from build123d import *

# Parameters (mm, degrees)
SKETCH1_W           = 8
SKETCH1_H           = 23
BOSS_EXTRUDE1_DEPTH = 3
SKETCH2_W           = 8
SKETCH2_H           = 3
BOSS_EXTRUDE2_DEPTH = 18
SKETCH3_R           = 1.75
CUT_EXTRUDE1_DEPTH  = 8
SKETCH4_R           = 1.75
CUT_EXTRUDE2_DEPTH  = 8


with BuildPart() as part:
    # Sketch1 → Boss-Extrude1 (new body)
    with BuildSketch(Plane.XY):
        with Locations((-48.217529248, 5.656933129)):
            Rectangle(SKETCH1_W, SKETCH1_H)
    extrude(amount=BOSS_EXTRUDE1_DEPTH)

    # Sketch2 → Boss-Extrude2 (add)
    with BuildSketch(Plane(origin=(0, 0, 0), x_dir=(-1, 0, 0), z_dir=(0, 0, -1))):
        with Locations((48.217529248, -4.343066871)):
            Rectangle(SKETCH2_W, SKETCH2_H)
    extrude(amount=BOSS_EXTRUDE2_DEPTH)

    # Sketch3 → Cut-Extrude1 (cut)
    with BuildSketch(Plane(origin=(0, -5.843066871, 0), x_dir=(-1, 0, 0), z_dir=(0, -1, 0))):
        with Locations(Location((48.217529248, 14, 0), (0, 0, 90))):
            Circle(SKETCH3_R)
    extrude(amount=-CUT_EXTRUDE1_DEPTH, mode=Mode.SUBTRACT)

    # Sketch4 → Cut-Extrude2 (cut)
    with BuildSketch(Plane.XY.offset(3)):
        with Locations((-48.217529248, 13.156933129)):
            Circle(SKETCH4_R)
    extrude(amount=-CUT_EXTRUDE2_DEPTH, mode=Mode.SUBTRACT)


solid = part.part
Build history of the part. All positions in model axes, mm. A direction names the side the tool comes from. Coordinates: 2 decimals unless noted, no trailing zeros. Order: outer loops, then holes, each group sorted by start corner. A loop starts at its lowest first (then second) coordinate and runs counter-clockwise, first axis right, second up. Notation, with made-up numbers: (61.5, 70) -> (111.5, 70) arc R14 ccw to (111.5, 81) -> close; hole circle Ø11 at (66.25, 53). An arc over 180 degrees is marked (long way). One line per item, written item: value.
(1) Probe line 1 (Z direction, x = -47.25, y = -1.75); line 2 (Y direction, x = -47.5, z = -5); line 3 (Z direction, x = -48, y = -3). List the from-to ranges inside material, lowest first. Write a range as [from, to].
Checked values:
line 1: [0, 3]
line 2: [-5.84, -2.84]
line 3: [-18, -15.74], [-12.26, 3]
(2) Mould opens along X. For faces 1 (the flat face through (-52.218, 0.5, 0.3)), 2 (the flat face through (-48, -4, -18)), 3 (the cylindrical face through (-46.482, -4.364, -13.772)) say: pulls with the +X half, pulls with the -X half, needs draft (parallel to the pull), parting line crosses it, or undercut.
Checked values:
face 1: pulls with the -X half
face 2: needs draft
face 3: undercut
(3) Slice it at B-B, the plane x = -48.5. List the corners of the cut face in (y, z).
Checked values:
outline: (-5.84, -18) -> (-2.84, -18) -> (-2.84, -15.73) -> (-5.84, -15.73) -> close; (-5.84, -12.27) -> (-2.84, -12.27) -> (-2.84, 0) -> (11.43, 0) -> (11.43, 3) -> (-5.84, 3) -> close; (14.88, 0) -> (17.16, 0) -> (17.16, 3) -> (14.88, 3) -> close
(4) Tool access for faces 4 (the cylindrical face through (-47.277, 14.633, 1.521)), 5 (the flat face through (-48, -2.843, -9)): list every direction of +Z, -Z, +X, -X, +Y, -Y with a clear straight run to the whole face (end or side of a thin tool).
Checked values:
face 4: +Z, -Z
face 5: -Z, +X, -X, +Y
(5) Slice it at C-C, the plane x = -50.75. List the corners of the cut face in (y, z).
Checked values:
outline: (-5.84, -18) -> (-2.84, -18) -> (-2.84, 0) -> (17.16, 0) -> (17.16, 3) -> (-5.84, 3) -> close
(6) Slice it at D-D, the plane y = 15.75. List the corners of the cut face in (x, z), plus the area to 3 significant figures.
Checked values:
outline: (-52.22, 0) -> (-44.22, 0) -> (-44.22, 3) -> (-52.22, 3) -> close
area: 24.0 mm2
(7) Slice it at A-A, the plane z = -14. List the corners of the cut face in (x, y), plus the area to 3 significant figures.
Checked values:
outline: (-52.22, -5.84) -> (-49.97, -5.84) -> (-49.97, -2.84) -> (-52.22, -2.84) -> close; (-46.47, -5.84) -> (-44.22, -5.84) -> (-44.22, -2.84) -> (-46.47, -2.84) -> close
area: 13.5 mm2
(8) Drop flat-ended pins along their axis: pin 1 Ø4 at (x, y) = (-50, 3.5) entering from -Z; pin 2 Ø3 at (x, z) = (-48.5, -9.5) entering from +Y. Give the stop position or say it passes through.
Checked values:
pin 1: z = 0
pin 2: y = -2.84
